Work out the finished part from the listing and answer in its coordinate system (mm). Round coordinates to 2 decimals unless told otherwise and drop trailing zeros. Return JSON: item names as keys, results as strings.
from build123d import *

# Parameters (mm, degrees)
SKIZZE1_W                       = 5
SKIZZE1_H                       = 15.5
GRUNDSTAB_DEPTH                 = 580
AUFSATZ_LINEAR_AUSTRAGEN2_DEPTH = 5
SKIZZE4_R                       = 3
SCHNITT_LINEAR_AUSTRAGEN1_DEPTH = 581.228618736


with BuildPart() as part:
    # Skizze1 → GrundStab (new body)
    with BuildSketch(Plane.XY):
        with Locations((2.5, 7.75)):
            Rectangle(SKIZZE1_W, SKIZZE1_H)
    extrude(amount=GRUNDSTAB_DEPTH)

    # Skizze3 → Aufsatz-Linear austragen2 (add, through all)
    with BuildSketch(Plane.ZY):
        Polygon((0, 7.75), (-80, 2), (-80, 0), (0, 0), align=None)
    extrude(amount=-AUFSATZ_LINEAR_AUSTRAGEN2_DEPTH)

    # Skizze4 → Schnitt-Linear austragen1 (cut, through all)
    with BuildSketch(Plane.ZY):
        with Locations((572, 7.75)):
            Circle(SKIZZE4_R)
        with Locations((562, 7.75)):
            Circle(SKIZZE4_R)
        with Locations((552, 7.75)):
            Circle(SKIZZE4_R)
        with Locations((540, 7.75)):
            Circle(SKIZZE4_R)
        with Locations((528, 7.75)):
            Circle(SKIZZE4_R)
        with Locations((516, 7.75)):
            Circle(SKIZZE4_R)
        with Locations((504, 7.75)):
            Circle(SKIZZE4_R)
        with Locations((488, 7.75)):
            Circle(SKIZZE4_R)
        with Locations((472, 7.75)):
            Circle(SKIZZE4_R)
        with Locations((456, 7.75)):
            Circle(SKIZZE4_R)
        with Locations((440, 7.75)):
            Circle(SKIZZE4_R)
        with Locations((424, 7.75)):
            Circle(SKIZZE4_R)
        with Locations((408, 7.75)):
            Circle(SKIZZE4_R)
        with Locations((392, 7.75)):
            Circle(SKIZZE4_R)
        with Locations((372, 7.75)):
            Circle(SKIZZE4_R)
        with Locations((352, 7.75)):
            Circle(SKIZZE4_R)
        with Locations((332, 7.75)):
            Circle(SKIZZE4_R)
        with Locations((312, 7.75)):
            Circle(SKIZZE4_R)
        with Locations((292, 7.75)):
            Circle(SKIZZE4_R)
    extrude(amount=-SCHNITT_LINEAR_AUSTRAGEN1_DEPTH, mode=Mode.SUBTRACT)


solid = part.part
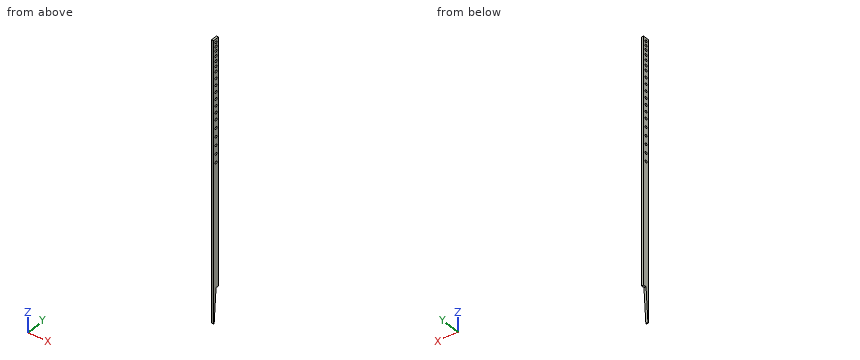
1) Section A-A (x = 3.75) is taken. Count the separate pieces of the cut face and the enclosed holes in it, and give its area (3 significant figures).
Verdict:
{"separate pieces": "1", "enclosed holes": "19", "area": "8,840 mm2"}
2) Find the intervals of material crossed by L1, parallel to Y at x = 4, z = 528; L2, parallel to Z at x = 1.45, y = 11; L3, parallel to Y at x = 0.5, z = 518.5, in increasing order.
Verdict:
{"L1": "y = 0 to 4.75, 10.75 to 15.5", "L2": "z = 0 to 580", "L3": "y = 0 to 6.09, 9.41 to 15.5"}
3) Flat-ended cylindrical pins translate along their axes: pin 1 (1 mm diameter, centred on y = 9, z = 383.5, fed in from -X); pin 2 (1.5 mm diameter, centred on x = 3.5, y = 14, fed in from -Z). Find the tip coordinate at first contact, or state that the pin passes through.
Verdict:
{"pin 1": "stops at x = 0", "pin 2": "stops at z = 0"}
